The listing builds one solid part. Answer for the finished solid, in the listing's coordinates (mm). Face numbers are marked on the shaded views. A direction names the side the tool comes from. Round coordinates to 2 decimals unless told otherwise and drop trailing zeros. Loops run counter-clockwise (first coordinate to the right, second up) from the corner with the lowest first, then second, coordinate; pieces in that order, holes last. Notation, with made-up numbers: (-24, 24) -> (-18, 24) arc R25 cw to (-18, 37) -> close; hole circle Ø7 at (-32, 83.5). An arc over 180 degrees is marked (long way). Write each question's results on one line, items separated by ' | '. Start each with the question number.
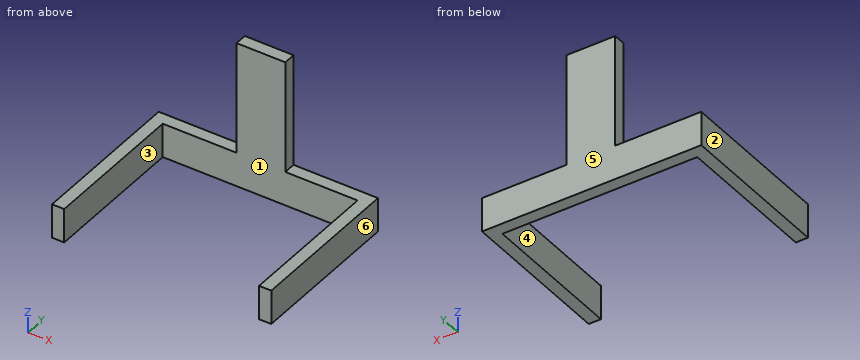
from build123d import *

# Parameters (mm, degrees)
F0_W     = 12.7
F0_H     = 38.1
F1_DEPTH = 3.175
F3_DEPTH = 3.175
F4_W     = 3.175
F4_H     = 8.89
F5_DEPTH = 38.1


with BuildPart() as f1:
    # F0 (on Front) → F1 (new body)
    with BuildSketch(Plane.XZ):
        Rectangle(F0_W, F0_H)
    extrude(amount=F1_DEPTH)

    # F2 (on face) → F3 (join)
    with BuildSketch(Plane.XZ.offset(3.175)):
        Polygon((-4.688735, -19.05), (6.35, -19.05), (28.369022, -19.05), (28.369022, -10.16), (3.864823, -10.16), (-6.35, -10.16), (-28.780978, -10.16), (-28.780978, -19.05), align=None)
    extrude(amount=-F3_DEPTH)

    # F4 (on face) → F5 (join)
    with BuildSketch(Plane.XZ.offset(3.175)):
        with Locations((-27.193478, -14.605)):
            Rectangle(F4_W, F4_H)
        with Locations((26.781522, -14.605)):
            Rectangle(F4_W, F4_H)
    extrude(amount=F5_DEPTH)


solid = f1.part
Item 1: The part is cut by section C-C, the plane x = -14.5. Give the vertices of the cut face in (y, z) (3 decimals), plus the area to 3 significant figures.
Item 2: For the marked faces 1 and 2, determine the directions among +Z, -Z, +X, -X, +Y, -Y from which every point of the face is accessible in a straight line to the end or side of a thin tool.
Item 3: The part is cut by section D-D, the plane z = 10. Give the vertices of the cut face in (x, y) (3 decimals).
Item 4: Determine the mould class of the marked faces 3, 4, 5 and 6 for opening direction X: +X half, -X half, draft (parallel to the pull), parting line (faces both ways), or undercut.
Item 5: The part is cut by section B-B, the plane z = -14.5. Give the vertices of the cut face in (x, y) (3 decimals), plus the area to 3 significant figures.
Item 6: The part is cut by section A-A, the plane y = -21.5. Give the vertices of the cut face in (x, z).
Item 7: Each of these flat-tipped pins is pushed along its axis until it touches: pin 1 Ø1 at (y, z) = (-1.5, 8) entering from -X; pin 2 Ø12 at (x, y) = (-20.5, -25) entering from +Z; pin 3 Ø1.6 at (y, z) = (-1.5, 2) entering from +X. Where does it stop, or does it pass through?
Item 8: Straight lines are drawn through the part: L1, parallel to X at y = -36, z = -15; L2, parallel to Z at x = 25.5, y = -31.5; L3, parallel to Y at x = 1.5, z = -9 (3 decimals). For each, find the intervals that lie inside material, in ascending order. Write a range as [from, to].
Report:
1) outline: (-3.175, -19.05) -> (0, -19.05) -> (0, -10.16) -> (-3.175, -10.16) -> close | area: 28.2 mm2
2) face 1: +Z, -Z, -Y | face 2: +Z, -Z, -X, +Y, -Y
3) outline: (-6.35, -3.175) -> (6.35, -3.175) -> (6.35, 0) -> (-6.35, 0) -> close
4) face 3: undercut | face 4: undercut | face 5: draft | face 6: +X half
5) outline: (-28.781, -41.275) -> (-25.606, -41.275) -> (-25.606, -3.175) -> (25.194, -3.175) -> (25.194, -41.275) -> (28.369, -41.275) -> (28.369, 0) -> (-28.781, 0) -> close | area: 423 mm2
6) outline: (-28.78, -19.05) -> (-25.61, -19.05) -> (-25.61, -10.16) -> (-28.78, -10.16) -> close; (25.19, -19.05) -> (28.37, -19.05) -> (28.37, -10.16) -> (25.19, -10.16) -> close
7) pin 1: stops at x = -6.35 | pin 2: stops at z = -10.16 | pin 3: stops at x = 6.35
8) L1: x = [-28.78, -25.61], [25.19, 28.37] | L2: z = [-19.05, -10.16] | L3: y = [-3.175, 0]
